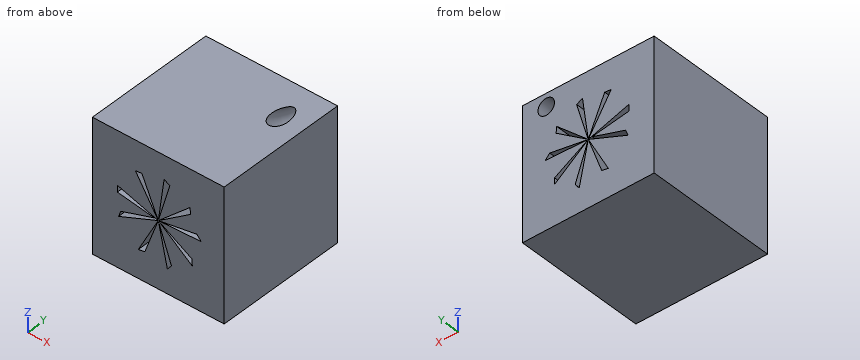
```python
from build123d import *

# Parameters (mm, degrees)
F0_W     = 25.4
F0_H     = 25.4
F1_DEPTH = 25.4
F2_R     = 1.5875


with BuildPart() as f1:
    # F0 (on Front) → F1 (new body)
    with BuildSketch(Plane.XZ):
        with Locations((12.7, 12.7)):
            Rectangle(F0_W, F0_H)
        with BuildLine():
            ThreePointArc((12.705212, 12.717705), (12.709806, 12.715636), (12.713669, 12.712402))
            Line((12.713669, 12.712402), (18.839256, 18.270461))
            Line((18.839256, 18.270461), (18.888431, 17.001414))
            Line((18.888431, 17.001414), (12.715155, 12.710534))
            ThreePointArc((12.715155, 12.710534), (12.717086, 12.706979), (12.718196, 12.703089))
            Line((12.718196, 12.703089), (20.130168, 13.961521))
            Line((20.130168, 13.961521), (20.983567, 13.020983))
            Line((20.983567, 13.020983), (12.718443, 12.700715))
            ThreePointArc((12.718443, 12.700715), (12.718453, 12.700357), (12.718457, 12.7))
            ThreePointArc((12.718457, 12.7), (12.717813, 12.695167), (12.715926, 12.690672))
            Line((12.715926, 12.690672), (19.202692, 8.891313))
            Line((19.202692, 8.891313), (19.251904, 7.621313))
            Line((19.251904, 7.621313), (12.714587, 12.688693))
            ThreePointArc((12.714587, 12.688693), (12.71083, 12.685055), (12.706202, 12.682617))
            Line((12.706202, 12.682617), (15.232591, 5.601773))
            Line((15.232591, 5.601773), (14.454533, 4.598018))
            Line((14.454533, 4.598018), (12.703906, 12.681962))
            ThreePointArc((12.703906, 12.681962), (12.698736, 12.681587), (12.693665, 12.682665))
            Line((12.693665, 12.682665), (10.106196, 5.601773))
            Line((10.106196, 5.601773), (8.836196, 5.365729))
            Line((8.836196, 5.365729), (12.691398, 12.683671))
            ThreePointArc((12.691398, 12.683671), (12.686331, 12.687598), (12.682914, 12.693021))
            Line((12.682914, 12.693021), (5.025776, 9.565228))
            Line((5.025776, 9.565228), (5.493536, 10.745948))
            Line((5.493536, 10.745948), (11.965962, 12.817308))
            Line((11.965962, 12.817308), (4.806211, 13.961521))
            Line((4.806211, 13.961521), (4.806211, 15.231521))
            Line((4.806211, 15.231521), (12.682425, 12.705636))
            ThreePointArc((12.682425, 12.705636), (12.685413, 12.711307), (12.69016, 12.715615))
            Line((12.69016, 12.715615), (12.515285, 12.993107))
            Line((12.515285, 12.993107), (8.280237, 19.713287))
            Line((8.280237, 19.713287), (9.544288, 19.836069))
            Line((9.544288, 19.836069), (12.692535, 12.71688))
            ThreePointArc((12.692535, 12.71688), (12.697419, 12.718275), (12.702499, 12.718287))
            Line((12.702499, 12.718287), (13.82232, 20.913459))
            Line((13.82232, 20.913459), (14.940951, 20.312158))
            Line((14.940951, 20.312158), (12.705212, 12.717705))
        make_face(mode=Mode.SUBTRACT)
    extrude(amount=F1_DEPTH)

    # F2 (on Front) → F3 (revolve, cut)
    with BuildSketch(Plane.XZ):
        with Locations((20.805778, 22.889411)):
            Circle(F2_R)
    revolve(axis=Axis((14.381558, 0, 35.589411), (1, 0, 0)), mode=Mode.SUBTRACT)


solid = f1.part
```
Check sheet for the modelled part. Datum: model origin and axes. Units: mm. Give positions to 0.01 mm unless a question says otherwise; leave off trailing zeros. Write each loop counter-clockwise with the first axis right and the second up, starting at its lowest first coordinate (ties: lowest second). Pieces come first, ordered by that corner, then holes. Notation, with made-up numbers: (64.5, -26) -> (76.5, -26) arc R17 ccw to (76.5, 2) -> close; hole circle Ø1 at (-9, 30.5). An arc over 180 degrees is marked (long way). Use CSV: the item, a comma, the result in double quotes. Start each with the question number.
Q1. Cross-section at A-A on z = 10. Enter the section's corners in (x, y), and give its area (3 significant figures).
Q2. Cross-section at C-C on z = 7. Enter the section's corners in (x, y), and give its area (3 significant figures).
Q3. Scan lines: line 1 along X through (y, z) = (-11.5, 15.5); line 2 along Z through (x, y) = (8.5, -1); line 3 along X through (y, z) = (-21.5, 16.5). Record each from-to range of solid material in increasing order.
Q4. Cross-section at B-B on x = 11.5. Enter the section's corners in (y, z).
Working result:
1,outline,"(0, -25.4) -> (5.2, -25.4) -> (5.2, 0) -> (0, 0) -> close; (6.09, -25.4) -> (11.28, -25.4) -> (11.28, 0) -> (6.09, 0) -> close; (11.71, -25.4) -> (13.28, -25.4) -> (13.28, 0) -> (11.71, 0) -> close; (13.66, -25.4) -> (16.18, -25.4) -> (16.18, 0) -> (13.66, 0) -> close; (17.31, -25.4) -> (25.4, -25.4) -> (25.4, 0) -> (17.31, 0) -> close"
1,area,"573 mm^2"
2,outline,"(0, -25.4) -> (9.7, -25.4) -> (9.7, 0) -> (0, 0) -> close; (10.62, -25.4) -> (13.93, -25.4) -> (13.93, 0) -> (10.62, 0) -> close; (14.73, -25.4) -> (25.4, -25.4) -> (25.4, 0) -> (14.73, 0) -> close"
2,area,"601 mm^2"
3,line 1,"x = 0 to 10.94, 11.46 to 13.08, 13.52 to 15.79, 16.73 to 25.4"
3,line 2,"z = 0 to 10.98, 11.71 to 13.37, 14.05 to 19.36, 19.73 to 25.4"
3,line 3,"x = 0 to 10.31, 11.02 to 13.22, 13.82 to 16.89, 18.17 to 25.4"
4,outline,"(-25.4, 0) -> (0, 0) -> (0, 9.42) -> (-25.4, 9.42) -> close; (-25.4, 10.42) -> (0, 10.42) -> (0, 12.21) -> (-25.4, 12.21) -> close; (-25.4, 12.67) -> (0, 12.67) -> (0, 12.89) -> (-25.4, 12.89) -> close; (-25.4, 13.08) -> (0, 13.08) -> (0, 14.6) -> (-25.4, 14.6) -> close; (-25.4, 15.41) -> (0, 15.41) -> (0, 25.4) -> (-25.4, 25.4) -> close"
